The drawing under review shows one solid part. Ordinate dimensions are in mm from its lowest x, y, z. Coordinates: 2 decimals unless noted, no trailing zeros. Write each loop counter-clockwise with the first axis right and the second up, starting at its lowest first coordinate (ties: lowest second). Pieces come first, ordered by that corner, then holes. Notation, with made-up numbers: (26, 55.25) - (74, 55.25) arc R27 cw to (74, 72.25) - close; hole circle Ø2 at (29, 39). An arc over 180 degrees is marked (long way). Put each result on its own line as item: value. Start each with the question number.
Item 1: To check wall thickness, follow L1, parallel to Y at x = 13, z = 3; L2, parallel to X at y = 18, z = 4.25; L3, parallel to Y at x = 17.5, z = 6.5. State the ranges of each line that lie inside material, in increasing order. Write a range as [from, to].
Item 2: Consider section A-A on x = 12.5. Give the boundary of the cut face in (y, z), then the cut area to 3 significant figures.
Item 3: Consider section C-C on z = 9.25. Give the boundary of the cut face in (x, y) (3 decimals).
Item 4: Consider section B-B on z = 7.75. Give the boundary of the cut face in (x, y) (3 decimals).
Item 5: For pin 1 (1.5 mm diameter, centred on x = 3, z = 2.5, fed in from +Y); pin 2 (1 mm diameter, centred on x = 21, y = 13.5, fed in from -Z); pin 3 (5 mm diameter, centred on x = 19.5, z = 3.5, fed in from -Y), all flat-tipped, find the tip position at first contact; note any pin that passes through.
Item 6: Mouldability with a two-part tool opening along X and no side actions: class the marked faces 1, 2 and 3 as pulls with the +X half, pulls with the -X half, needs draft (parallel to the pull), parting line crosses it, or undercut.
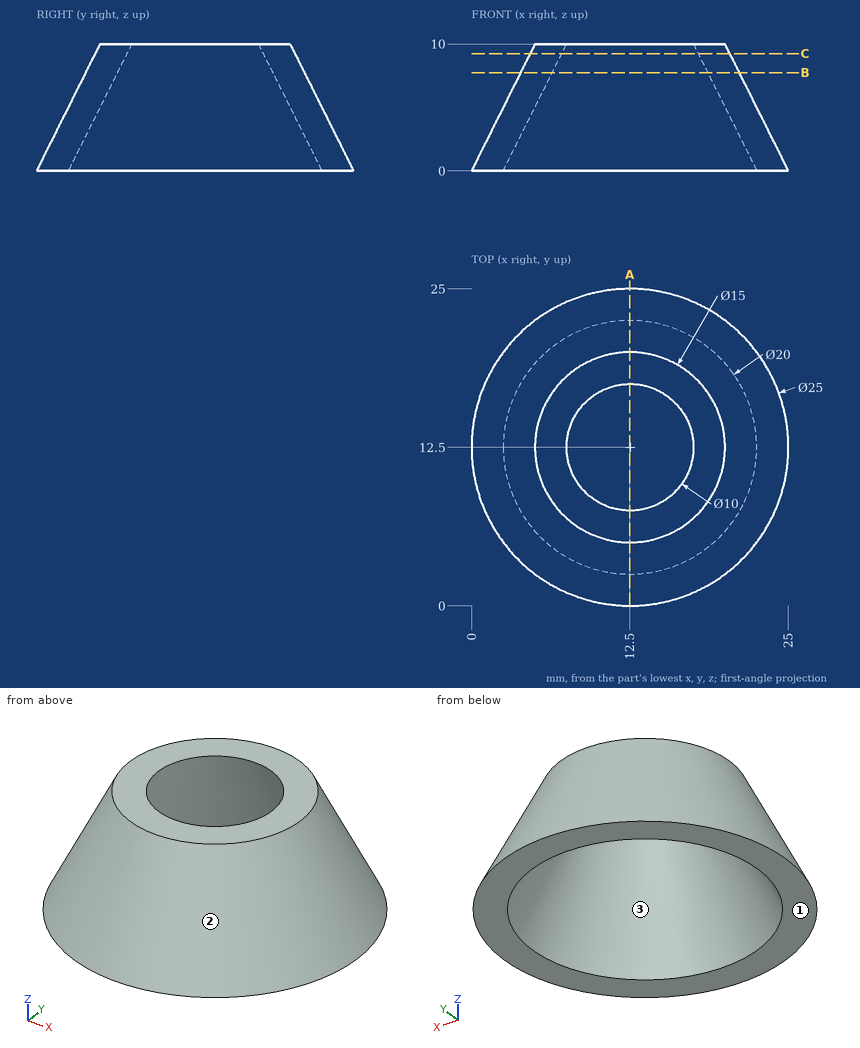
Report:
1. L1: [1.51, 4.01], [20.99, 23.49]
1. L2: [3.7, 6.86], [18.14, 21.3]
1. L3: [4.72, 7.97], [17.03, 20.28]
2. outline: (0, 0) - (2.5, 0) - (7.5, 10) - (5, 10) - close; (17.5, 10) - (22.5, 0) - (25, 0) - (20, 10) - close
2. area: 50.0 mm²
3. outline: circle Ø15.75 at (12.5, 12.5); hole circle Ø10.75 at (12.5, 12.5)
4. outline: circle Ø17.25 at (12.5, 12.5); hole circle Ø12.25 at (12.5, 12.5)
5. pin 1: y = 19.75
5. pin 2: z = 1.88
5. pin 3: y = 2.11
6. face 1: needs draft
6. face 2: parting line crosses it
6. face 3: undercut
